from build123d import *

# Parameters (mm, degrees)
SKETCH2_R           = 36.7
BOSS_EXTRUDE1_DEPTH = 11
SKETCH5_R           = 14.1
CUT_EXTRUDE1_DEPTH  = 4.5
BOSS_EXTRUDE2_START = 10
SKETCH7_R           = 36.7
SKETCH7_R_2         = 31.7
BOSS_EXTRUDE2_DEPTH = 10
CIRPATTERN1_COUNT   = 6


with BuildPart() as part:
    # Sketch2 → Boss-Extrude1 (new body)
    with BuildSketch(Plane(origin=(0, 0, 0), x_dir=(1, 0, 0), z_dir=(0, 1, 0))):
        with Locations(Location((0, 0, 0), (0, 0, 270))):
            Circle(SKETCH2_R)
    extrude(amount=BOSS_EXTRUDE1_DEPTH)

    # Sketch3 → Cut-Revolve1 (revolve, cut)
    with BuildSketch(Plane(origin=(0, 0, 0), x_dir=(0, 0, -1), z_dir=(1, 0, 0))):
        Polygon((26.8, 11), (26.8, 9.3), (25.9, 0.5), (25.9, 0), (23.8, 0), (23.8, 11), align=None)
    cut_revolve1 = revolve(axis=Axis((0, 0, -23.8), (0, 1, 0)), mode=Mode.SUBTRACT)

    # Sketch5 → Cut-Extrude1 (cut)
    with BuildSketch(Plane.XZ):
        with Locations(Location((0, 0, 0), (0, 0, 270))):
            Circle(SKETCH5_R)
    extrude(amount=-CUT_EXTRUDE1_DEPTH, mode=Mode.SUBTRACT)

    # Sketch7 → Boss-Extrude2 (add)
    with BuildSketch(Plane.XZ.offset(BOSS_EXTRUDE2_START)):
        with Locations(Location((0, 0, 0), (0, 0, 270))):
            Circle(SKETCH7_R)
        with Locations(Location((0, 0, 0), (0, 0, 270))):
            Circle(SKETCH7_R_2, mode=Mode.SUBTRACT)
    extrude(amount=-BOSS_EXTRUDE2_DEPTH)

    # CirPattern1: Cut-Revolve1 ×6 about axis
    cirpattern1_axis = Axis((0, 0, 0), (0, 1, 0))
    for i in range(1, CIRPATTERN1_COUNT):
        add(cut_revolve1.rotate(cirpattern1_axis, i * 360 / CIRPATTERN1_COUNT), mode=Mode.SUBTRACT)


solid = part.part
Build history of the part. All positions in model axes, mm. A direction names the side the tool comes from. Give positions to 0.01 mm unless a question says otherwise; leave off trailing zeros. Loops run counter-clockwise (first coordinate to the right, second up) from the corner with the lowest first, then second, coordinate; pieces in that order, holes last. Notation, with made-up numbers: (-28, -26.75) -> (20, -26.75) arc R26 ccw to (20, -2.75) -> close; hole circle Ø4 at (29, 53). An arc over 180 degrees is marked (long way). Answer in a Markdown table with one row per item.
Item 1: Tool access for faces 1 (the cylindrical face through (18.561, 0.246, -12.355)), 2 (the cylindrical face through (-5.4, 2.218, -13.025)), 3 (the cylindrical face through (23.586, 10.138, -12.291)): list every direction of +Z, -Z, +X, -X, +Y, -Y with a clear straight run to the whole face (end or side of a thin tool).
Findings below:
| item | result |
|---|---|
| face 1 | +Y, -Y |
| face 2 | -Y |
| face 3 | +Y |
Item 2: Flat gauge pins, fed straight in: P1, Ø3, axis at y = 0.5, z = -2, coming from the +X side; P2, Ø6.5, axis at x = 20.61, z = 11.9, coming from the -Y side; P3, Ø3, axis at y = 1, z = -14, coming from the -X side; P4, Ø8, axis at x = -2, y = -7.5, coming from the +Z side. Where does each tip first touch, or does it go through?
Findings below:
| item | result |
|---|---|
| P1 | stops at x = 36.7 |
| P2 | stops at y = 0 |
| P3 | stops at x = -34.51 |
| P4 | stops at z = 36.7 |
Item 3: Slice it at B-B on z = -11.9. Write the cut outline in (x, y), plus the area to 3 significant figures.
Findings below:
| item | result |
|---|---|
| outline | (-34.72, -10) -> (-29.38, -10) -> (-29.38, 0) -> (-22.71, 0) -> (-22.71, 0.5) -> (-23.61, 9.3) -> (-23.61, 11) -> (-34.72, 11) -> close; (-18.51, 0) -> (-7.56, 0) -> (-7.56, 4.5) -> (7.56, 4.5) -> (7.56, 0) -> (18.51, 0) -> (18.51, 0.5) -> (17.61, 9.3) -> (17.61, 11) -> (-17.61, 11) -> (-17.61, 9.3) -> (-18.51, 0.5) -> close; (22.71, 0) -> (29.38, 0) -> (29.38, -10) -> (34.72, -10) -> (34.72, 11) -> (23.61, 11) -> (23.61, 9.3) -> (22.71, 0.5) -> close |
| area | 688 mm² |
Item 4: Slice it at D-D on x = -29.5. Write the cut outline in (y, z).
Findings below:
| item | result |
|---|---|
| outline | (-10, -21.83) -> (11, -21.83) -> (11, 21.83) -> (-10, 21.83) -> (-10, 11.6) -> (0, 11.6) -> (0, -11.6) -> (-10, -11.6) -> close |
Item 5: Slice it at C-C on z = 23.8. Write the cut outline in (x, y).
Findings below:
| item | result |
|---|---|
| outline | (-27.94, -10) -> (-20.94, -10) -> (-20.94, 0) -> (-2.1, 0) -> (-2.1, 0.5) -> (-3, 9.3) -> (-3, 11) -> (-27.94, 11) -> close; (2.1, 0) -> (20.94, 0) -> (20.94, -10) -> (27.94, -10) -> (27.94, 11) -> (3, 11) -> (3, 9.3) -> (2.1, 0.5) -> close |
Item 6: Slice it at A-A on y = 6. Write the cut outline in (x, z) (1 decimal), plus the area to 3 significant figures.
Findings below:
| item | result |
|---|---|
| outline | circle Ø73.4 at (0, 0); hole circle Ø5.3 at (-20.6, -11.9); hole circle Ø5.3 at (-20.6, 11.9); hole circle Ø5.3 at (0, -23.8); hole circle Ø5.3 at (0, 23.8); hole circle Ø5.3 at (20.6, -11.9); hole circle Ø5.3 at (20.6, 11.9) |
| area | 4,100 mm² |
Item 7: Mould opens along X. For faces 4 (the cylindrical face through (22.66, 0.25, 12.36)), 5 (the flat face through (-11, -10, 30)) say: pulls with the +X half, pulls with the -X half, needs draft (parallel to the pull), parting line crosses it, or undercut.
Findings below:
| item | result |
|---|---|
| face 4 | undercut |
| face 5 | needs draft |
Item 8: Probe line 1 along X through (y, z) = (9.95, -11.9); line 2 along X through (y, z) = (3.5, -11.5); line 3 along Z through (x, y) = (-21.5, 4.5). List the from-to ranges inside material, lowest first. Write a range as [from, to].
Findings below:
| item | result |
|---|---|
| line 1 | x = [-34.72, -23.61], [-17.61, 17.61], [23.61, 34.72] |
| line 2 | x = [-34.85, -22.98], [-18.24, -8.16], [8.16, 18.24], [22.98, 34.85] |
| line 3 | z = [-29.74, -14.25], [-9.55, 9.55], [14.25, 29.74] |
